Autodesk Inventor part; units mm, degrees
ref_plane "YZ Plane" through (0, 0, 0) normal (1, 0, 0) x (0, 1, 0)
ref_plane "XZ Plane" through (0, 0, 0) normal (0, 1, 0) x (-1, 0, 0)
ref_plane "XY Plane" through (0, 0, 0) normal (0, 0, 1) x (1, 0, 0)
sketch "Esquisse1" plane through (0, 0, 0) normal (0, 1, 0) x (-1, 0, 0)
  circle A0 centre (0, 0) radius 2.5
  line L0 (0.75, -2.3848) -> (-0.75, -2.3848)
  line L1 (-0.75, -2.3848) -> (-0.75, -3.3848)
  line L2 (-0.75, -3.3848) -> (0.75, -3.3848)
  line L3 (0.75, -3.3848) -> (0.75, -2.3848)
  circle A1 centre (0, 0) radius 1.5
  dimension "d0" = 5
  dimension "d1" = 1.5
  dimension "d2" = 1
  dimension "d3" = 3
extrude "Extrusion1" add sketch "Esquisse1" along normal blind 9
sketch "Esquisse2" plane through (0, 0, 0) normal (0, -1, 0) x (1, 0, 0)
  circle A0 centre (0, 0) radius 1.5
  line L0 (-0.75, -3.3848) -> (-0.75, -2.3848)
  line L1 (0.75, -3.3848) -> (-0.75, -3.3848)
  line L2 (0.75, -2.3848) -> (0.75, -3.3848)
  arc A1 (0.75, -2.3848) -> (-0.75, -2.3848) centre (0, 0) ccw
  line L3 (2.5, 2.5) -> (-2.5, 2.5)
  line L4 (-2.5, 2.5) -> (-2.5, -3.3848)
  line L5 (-2.5, -3.3848) -> (2.5, -3.3848)
  line L6 (2.5, -3.3848) -> (2.5, 2.5)
  arc A2 (0.75, -2.3848) -> (-0.75, -2.3848) centre (0, 0) ccw
extrude "Extrusion2" add sketch "Esquisse2" along normal blind 1
sketch "Esquisse3" plane through (0, 0, 0) normal (0, 0, 1) x (1, 0, 0)
  circle A0 centre (0, 1.5) radius 1
  line L0 (1.5, -1) -> (-1.5, -1)
  point P0 (0, 0)
  dimension "d8" = 2
  dimension "d9" = 2.5
extrude "Extrusion3" cut sketch "Esquisse3" along normal up to surface
sketch "Esquisse4" plane through (0, 0, 0) normal (1, 0, 0) x (0, 1, 0)
  line L0 (0, 2.5) -> (9, 2.5)
  line L1 (9, 2.5) -> (7, -3.3848)
  line L2 (0, -3.3848) -> (9, -3.3848)
  line L3 (9, 2.5) -> (9, -3.3848)
  line L4 (7, -3.3848) -> (9, -3.3848)
  point P0 (0, 0)
  dimension "d13" = 2
extrude "Extrusion4" cut sketch "Esquisse4" along normal mid plane 6
properties part number "tige_ejection_douille"
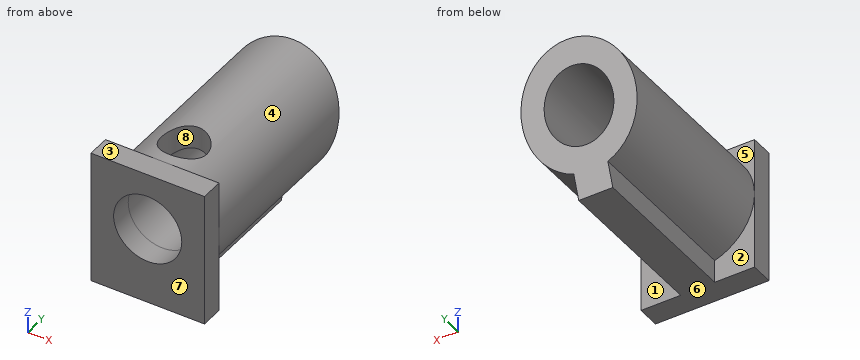
Input: part model. Units: mm. Frame: model coordinates. Face numbers are marked on the shaded views. A direction names the side the tool comes from. Give positions to 0.01 mm unless a question says otherwise; leave off trailing zeros. Order: outer loops, then holes, each group sorted by start corner. A loop starts at its lowest first (then second) coordinate and runs counter-clockwise, first axis right, second up. Notation, with made-up numbers: M 76.25,15 L 89.25,15 A24 ccw 89.25,36 Z; hole C 49,89 d4. An arc over 180 degrees is marked long. Return JSON: item names as keys, results as strings.
Item 1: First-contact query: P1, Ø1.9, axis at x = 1.5, z = -2.5, coming from the +Y side; P2, Ø2, axis at x = -1.5, z = 1, coming from the +Y side; P3, Ø0.5, axis at x = -1.5, z = -1.5, coming from the +Y side. Flat tips, straight axial feed; report the tip coordinate or a pass-through.
Solutions:
{"P1": "y = 7.62", "P2": "y = 8.83", "P3": "y = 7.73"}
Item 2: Cut plane C-C (x = -2.1). Return loops of the section in (y, z).
Solutions:
{"outline": "M -1,-3.38 L 0,-3.38 L 0,-1.36 L 7.69,-1.36 L 8.61,1.36 L 0,1.36 L 0,2.5 L -1,2.5 Z"}
Item 3: Ray query, probe 1 along X at (y, z) = (-0.3, 0); probe 2 along Z at (x, y) = (0, 4.5); probe 3 along Z at (x, y) = (-2, 1.5). Return the intervals inside material, ascending.
Solutions:
{"probe 1": "-2.5 to -1.5, 1.5 to 2.5", "probe 2": "-3.38 to -1.5, 1.5 to 2.5", "probe 3": "-1.5 to 1.5"}
Item 4: Pull-direction query (Y, two-part tool) for the marked faces 5, 6, 7 and 8; classes: +Y half, -Y half, draft (parallel to the pull), parting line (faces both ways), or undercut.
Solutions:
{"face 5": "+Y half", "face 6": "draft", "face 7": "-Y half", "face 8": "undercut"}
Item 5: Cut plane B-B (y = 5.5). Return loops of the section in (x, z), then the cut area to 3 significant figures.
Solutions:
{"outline": "M -0.75,-3.38 L 0.75,-3.38 L 0.75,-2.38 A2.5 ccw long -0.75,-2.38 Z; hole C 0,0 d3", "area": "14.0 mm^2"}
Item 6: Access query for the marked faces 1, 2, 3 and 4. Directions: +Z, -Z, +X, -X, +Y, -Y. A direction counts if a zero-diameter tool reaches every point of the face in a straight line with its end or side. Return the directions, or none.
Solutions:
{"face 1": "-Z, +X, +Y", "face 2": "-Z, -X, +Y", "face 3": "+Z, +X, -X, +Y, -Y", "face 4": "+Y"}
Item 7: Cut plane A-A (z = 0.6). Return loops of the section in (x, y).
Solutions:
{"outline": "M -2.5,-1 L -1.37,-1 L -1.37,8.35 L -2.43,8.35 L -2.43,0 L -2.5,0 Z; M 1.37,-1 L 2.5,-1 L 2.5,0 L 2.43,0 L 2.43,8.35 L 1.37,8.35 Z"}
